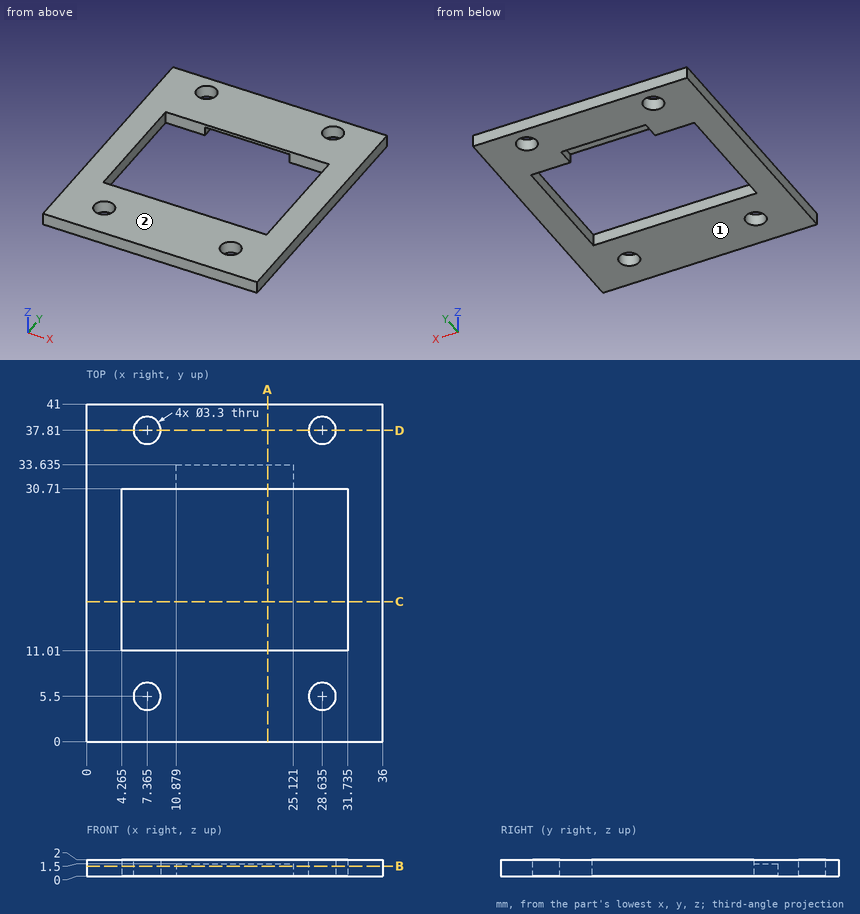
Could you check a few things on this drawing? It's one solid part, dimensions in mm from its lowest x, y, z. Coordinates: 2 decimals unless noted, no trailing zeros. Write each loop counter-clockwise with the first axis right and the second up, starting at its lowest first coordinate (ties: lowest second). Pieces come first, ordered by that corner, then holes. Notation, with made-up numbers: (54, 36) - (61, 36) arc R4 cw to (61, 42) - close; hole circle Ø11 at (54, 6.5). An arc over 180 degrees is marked (long way). Put each result on its own line as item: value. Start each with the question number.
Q1. I want a section at A-A on x = 22. Write out the boundary of the cut face in (y, z) (3 decimals), plus the area to 3 significant figures.
Q2. I want a section at D-D on y = 37.81. Write out the boundary of the cut face in (x, z) (3 decimals).
Q3. Thinking about a two-plate mould opening in Z: for the marked faces 1 and 2, which applies, pulls with the +Z half, pulls with the -Z half, needs draft (parallel to the pull), parting line crosses it, or undercut?
Q4. I'm going to push a flat-ended pin straight in: P1, Ø0.9, axis at x = 21.5, y = 32, coming from the -Z side. Where does the tip first touch, or does it pass through?
Q5. I want a section at C-C on y = 17. Write out the boundary of the cut face in (x, z) (3 decimals).
Q6. I want a section at B-B on z = 1.2. Write out the boundary of the cut face in (x, y) (3 decimals), plus the area to 3 significant figures.
Q7. Please list where these lines run through material, in increasing order: L1, parallel to X at y = 16, z = 1.95 (3 decimals); L2, parallel to X at y = 37.81, z = 1.4 (3 decimals); L3, parallel to Y at x = 25, z = 1.35 (3 decimals).
Checks:
1. outline: (0, 0) - (11.01, 0) - (11.01, 2) - (0, 2) - close; (30.71, 1.5) - (33.635, 1.5) - (33.635, 0) - (41, 0) - (41, 2) - (30.71, 2) - close
1. area: 38.2 mm²
2. outline: (0, 0) - (5.715, 0) - (5.715, 2) - (0, 2) - close; (9.015, 0) - (26.985, 0) - (26.985, 2) - (9.015, 2) - close; (30.285, 0) - (36, 0) - (36, 2) - (30.285, 2) - close
3. face 1: pulls with the -Z half
3. face 2: pulls with the +Z half
4. P1: z = 1.5
5. outline: (0, 0) - (4.265, 0) - (4.265, 2) - (0, 2) - close; (31.735, 0) - (36, 0) - (36, 2) - (31.735, 2) - close
6. outline: (0, 0) - (36, 0) - (36, 41) - (0, 41) - close; hole (4.265, 11.01) - (31.735, 11.01) - (31.735, 30.71) - (25.121, 30.71) - (25.121, 33.635) - (10.879, 33.635) - (10.879, 30.71) - (4.265, 30.71) - close; hole circle Ø3.3 at (7.365, 5.5); hole circle Ø3.3 at (7.365, 37.81); hole circle Ø3.3 at (28.635, 5.5); hole circle Ø3.3 at (28.635, 37.81)
6. area: 859 mm²
7. L1: 0 to 4.265, 31.735 to 36
7. L2: 0 to 5.715, 9.015 to 26.985, 30.285 to 36
7. L3: 0 to 11.01, 33.635 to 41
